from build123d import *

# Parameters (mm, degrees)
SKETCH1_W           = 16
SKETCH1_H           = 4.1
SKETCH1_W_2         = 4
SKETCH1_H_2         = 15.2
BOSS_EXTRUDE2_DEPTH = 3.7
FILLET1_R           = 10
FILLET2_R           = 10


with BuildPart() as part:
    # Sketch1 → Boss-Extrude2 (new body)
    with BuildSketch(Plane.XY):
        Polygon((-110.178290248, 0), (31.421709752, 0), (31.421709752, -59.4), (22.021709752, -59.4), (4.921709752, -47.383344891), (-83.678290248, -47.383344891), (-100.778290248, -59.4), (-110.178290248, -59.4), align=None)
        with BuildLine():
            Line((0.171709752, -21.7), (-78.928290248, -21.7))
            ThreePointArc((-78.928290248, -21.7), (-86.778290248, -13.85), (-78.928290248, -6))
            Line((-78.928290248, -6), (0.171709752, -6))
            ThreePointArc((0.171709752, -6), (8.021709752, -13.85), (0.171709752, -21.7))
        make_face(mode=Mode.SUBTRACT)
        with Locations((-23.078290248, -30.55)):
            Rectangle(SKETCH1_W, SKETCH1_H, mode=Mode.SUBTRACT)
        with Locations((-55.678290248, -30.55)):
            Rectangle(SKETCH1_W, SKETCH1_H, mode=Mode.SUBTRACT)
        with Locations((25.721709752, -41.9)):
            Rectangle(SKETCH1_W_2, SKETCH1_H_2, mode=Mode.SUBTRACT)
        with Locations((-104.478290248, -41.9)):
            Rectangle(SKETCH1_W_2, SKETCH1_H_2, mode=Mode.SUBTRACT)
    extrude(amount=BOSS_EXTRUDE2_DEPTH)

    # Fillet1
    fillet1_edges = [part.edges().sort_by_distance(p)[0] for p in [
        (-110.178290248, 0, 1.85),
        (31.421709752, 0, 1.85),
    ]]
    fillet(fillet1_edges, radius=FILLET1_R)

    # Fillet2
    fillet2_edges = [part.edges().sort_by_distance(p)[0] for p in [
        (4.921709752, -47.383344891, 1.85),
        (-83.678290248, -47.383344891, 1.85),
    ]]
    fillet(fillet2_edges, radius=FILLET2_R)


solid = part.part
The listing builds one solid part. Answer for the finished solid, in the listing's coordinates (mm). A direction names the side the tool comes from. Give positions to 0.01 mm unless a question says otherwise; leave off trailing zeros. Write each loop counter-clockwise with the first axis right and the second up, starting at its lowest first coordinate (ties: lowest second). Pieces come first, ordered by that corner, then holes. Notation, with made-up numbers: (-23.75, 38.25) - (-6.75, 38.25) arc R23 ccw to (-6.75, 64.25) - close; hole circle Ø9 at (67.25, 71.5). An arc over 180 degrees is marked (long way). One line per question, with ' | ' between items. Start each with the question number.
1. Section B-B, the plane y = -13.85 is taken. Determine the outline of the cut face in (x, z).
2. Section C-C, the plane z = 1.3 is taken. Count the separate pieces of the cut face and the enclosed holes in it, then the cut area to 3 significant figures.
3. Straight lines are drawn through the part: line 1 (X direction, y = -39, z = 2.6); line 2 (Y direction, x = -59, z = 1.1); line 3 (X direction, y = -32, z = 3.55). For each, find the intervals that lie inside material, in ascending order.
4. Given P1, Ø1.8, axis at x = -55.5, z = 1.5, coming from the -Y side, flat-ended and moving along its own axis, determine where the tip first touches the part or whether it passes through.
5. For faces 4 (the face through (-63.678, -31, 2)), 5 (the face through (28.415, -2.852, 1.876)), determine the directions among +Z, -Z, +X, -X, +Y, -Y from which every point of the face is accessible in a straight line to the end or side of a thin tool.
6. Determine the mould class of faces 1 (the face through (14.867, -54.372, 1.824)), 2 (the face through (23.722, -42, 2)), 3 (the face through (-38, -29, 3.7)) for opening direction Y: +Y half, -Y half, draft (parallel to the pull), parting line (faces both ways), or undercut.
7. Section D-D, the plane y = -54.5 is taken. Determine the outline of the cut face in (x, z).
8. Section A-A, the plane x = -25 is taken. Determine the outline of the cut face in (y, z).
Result:
1) outline: (-110.18, 0) - (-86.78, 0) - (-86.78, 3.7) - (-110.18, 3.7) - close; (8.02, 0) - (31.42, 0) - (31.42, 3.7) - (8.02, 3.7) - close
2) separate pieces: 1 | enclosed holes: 5 | area: 5,410 mm2
3) line 1: x = -110.18 to -106.48, -102.48 to 23.72, 27.72 to 31.42 | line 2: y = -47.38 to -32.6, -28.5 to -21.7, -6 to 0 | line 3: x = -110.18 to -63.68, -47.68 to -31.08, -15.08 to 31.42
4) P1: stops at y = -47.38
5) face 4: +Z, -Z | face 5: +Z, -Z, +X, +Y
6) face 1: -Y half | face 2: undercut | face 3: draft
7) outline: (-110.18, 0) - (-93.81, 0) - (-93.81, 3.7) - (-110.18, 3.7) - close; (15.05, 0) - (31.42, 0) - (31.42, 3.7) - (15.05, 3.7) - close
8) outline: (-47.38, 0) - (-32.6, 0) - (-32.6, 3.7) - (-47.38, 3.7) - close; (-28.5, 0) - (-21.7, 0) - (-21.7, 3.7) - (-28.5, 3.7) - close; (-6, 0) - (0, 0) - (0, 3.7) - (-6, 3.7) - close
